```python
from build123d import *


with BuildPart() as part:
    # Esquisse1 → Bague exterieure (revolve)
    with BuildSketch(Plane.XY, mode=Mode.PRIVATE) as bague_exterieure_sk:
        with BuildLine():
            Line((0, 12), (0, 13.5))
            ThreePointArc((0, 13.5), (0.146446609, 13.853553391), (0.5, 14))
            Line((0.5, 14), (7.5, 14))
            ThreePointArc((7.5, 14), (7.853553391, 13.853553391), (8, 13.5))
            Line((8, 13.5), (8, 12))
            Line((8, 12), (5.5, 12))
            ThreePointArc((5.5, 12), (4, 12.5), (2.5, 12))
            Line((2.5, 12), (0, 12))
        make_face()
    revolve(bague_exterieure_sk.sketch.rotate(Axis((0, 0, 0), (1, 0, 0)), 90), axis=Axis((0, 0, 0), (1, 0, 0)))


solid = part.part
```
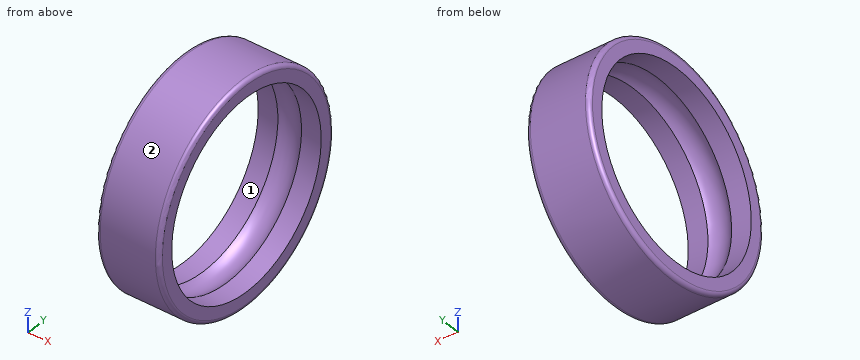
Part model, mm, in its own coordinate system. Face numbers are marked on the shaded views. Round coordinates to 2 decimals unless told otherwise and drop trailing zeros. Write each loop counter-clockwise with the first axis right and the second up, starting at its lowest first coordinate (ties: lowest second). Pieces come first, ordered by that corner, then holes. Notation, with made-up numbers: M 76,63 L 87,63 A21 cw 87,83 Z; hole C 26.5,74.25 d6. An arc over 180 degrees is marked long. Answer as CSV lines item,"result". Start each with the question number.
1) Band-saw the part on C-C (x = 6.25). List the corners of the cut face in (y, z).
2) Band-saw the part on D-D (x = 3.5). List the corners of the cut face in (y, z), then the cut area to 3 significant figures.
3) Mould opens along Z. For the marked faces 1 and 2 say: +Z half, -Z half, draft (parallel to the pull), parting line (faces both ways), or undercut.
4) Band-saw the part on A-A (z = 0). List the corners of the cut face in (x, y), then the cut area to 3 significant figures.
5) Drop flat-ended pins along their axis: pin 1 (1 mm diameter, centred on x = 3, z = -11, fed in from -Y); pin 2 (4 mm diameter, centred on x = 2.5, z = -3.5, fed in from +Y). Give the stop position or say it passes through.
6) Drill centre lines: L1, parallel to Y at x = 1.6, z = 0; L2, parallel to Y at x = 5.5, z = -4.5; L3, parallel to Z at x = 1, y = 4. Where is each one in solid material? Low to high.
Worked out:
1,outline,"C 0,0 d28; hole C 0,0 d24"
2,outline,"C 0,0 d28; hole C 0,0 d24.9"
2,area,"129 mm²"
3,face 1,"undercut"
3,face 2,"parting line"
4,outline,"M 0,-13.5 A0.5 ccw 0.5,-14 L 7.5,-14 A0.5 ccw 8,-13.5 L 8,-12 L 5.5,-12 A2.5 cw 2.5,-12 L 0,-12 Z; M 0,12 L 2.5,12 A2.5 cw 5.5,12 L 8,12 L 8,13.5 A0.5 ccw 7.5,14 L 0.5,14 A0.5 ccw 0,13.5 Z"
4,area,"29.7 mm²"
5,pin 1,"y = -9.26"
5,pin 2,"y = 13.92"
6,L1,"-14 to -12, 12 to 14"
6,L2,"-13.26 to -11.12, 11.12 to 13.26"
6,L3,"-13.42 to -11.31, 11.31 to 13.42"
